Geometry check sheet. Reference: the model listing, model coordinates, mm. A direction names the side the tool comes from. Round coordinates to 2 decimals unless told otherwise and drop trailing zeros. Write each loop counter-clockwise with the first axis right and the second up, starting at its lowest first coordinate (ties: lowest second). Pieces come first, ordered by that corner, then holes.
Autodesk Inventor part; units mm, degrees
ref_plane "YZ Plane" through (0, 0, 0) normal (1, 0, 0) x (0, 1, 0)
ref_plane "XZ Plane" through (0, 0, 0) normal (0, 1, 0) x (-1, 0, 0)
ref_plane "XY Plane" through (0, 0, 0) normal (0, 0, 1) x (1, 0, 0)
sketch "Sketch1" plane through (0, 0, 0) normal (0, 0, 1) x (1, 0, 0)
  line L0 (0, 0) -> (0, 110)
  line L1 (18, 130) -> (63, 130)
  line L2 (0, 0) -> (175, 0)
  line L3 (175, 0) -> (63, 130)
  line L4 (165, 0) -> (165, -10)
  line L5 (165, -10) -> (55, -10)
  line L6 (55, -10) -> (55, 0)
  line L7 (0, 110) -> (0, 130)
  line L8 (0, 130) -> (18, 130)
  dimension "d1" = 110
  dimension "d5" = 45
  dimension "d6" = 175
  dimension "d7" = 10
  dimension "d8" = 10
  dimension "d9" = 110
extrude "Extrusion1" add sketch "Sketch1" along normal blind 5
fillet "Fillet1" radius 2.5 2 edges at (119, 65, 5) (119, 65, 0)
properties part number "vertikal stab"
1. Depth check by flat-ended pin: pin 1 Ø1.5 at (x, y) = (101.5, 12) entering from -Z. Enter the tip coordinate at first touch or a pass-through.
2. Scan lines: line 1 along Y through (x, z) = (21, 3.5); line 2 along X through (y, z) = (-1.5, 2.75); line 3 along X through (y, z) = (54, 3.9). Record each from-to range of solid material in increasing order.
3. Access from +Z, -Z, +X, -X, +Y, -Y to the whole of each face (thin tool, end or side, straight path). Record for faces 4 (the face through (55, -5, 2)), 5 (the face through (170, 0, 2)), 6 (the face through (66, 45, 0)).
4. Release check for a two-part mould opening along Y. For faces 1 (the face through (27, 0, 2)), 2 (the face through (165, -5, 2)), 3 (the face through (117, 66.3, 0.8)) record: +Y half, -Y half, draft (parallel to the pull), parting line (faces both ways), or undercut.
5. Section check A-A (z = 3.55). Record the cut outline in (x, y).
Results below:
1. pin 1: stops at z = 0
2. line 1: y = 0 to 130
2. line 2: x = 55 to 165
2. line 3: x = 0 to 127.91
3. face 4: +Z, -Z, -X, -Y
3. face 5: +Z, -Z, +X, -Y
3. face 6: -Z, +X, -X, +Y, -Y
4. face 1: -Y half
4. face 2: draft
4. face 3: +Y half
5. outline: (0, 0) - (55, 0) - (55, -10) - (165, -10) - (165, 0) - (174.7, 0) - (62.7, 130) - (0, 130) - close
